The drawing under review shows one solid part. Ordinate dimensions are in mm from its lowest x, y, z. Round coordinates to 2 decimals unless told otherwise and drop trailing zeros. Write each loop counter-clockwise with the first axis right and the second up, starting at its lowest first coordinate (ties: lowest second). Pieces come first, ordered by that corner, then holes. Notation, with made-up numbers: (-5, -13) -> (44, -13) arc R30 cw to (44, 26) -> close; hole circle Ø7 at (-3, 3). An arc over 180 degrees is marked (long way). Write item = value, one per line. Start each with the question number.
Item 1: Add section B-B, the plane z = 150. State the section outline as (x, y) points.
Item 2: For pin 1 Ø13.5 at (x, z) = (20, 150) entering from -Y, flat-tipped, find the tip position at first contact; note if it passes through.
Item 3: To check wall thickness, follow L1, parallel to Z at x = 20, y = 5.25; L2, parallel to X at y = 4.5, z = 150; L3, parallel to Z at x = 13.5, y = 6.75. State the ranges of each line that lie inside material, in increasing order.
Item 4: Add section A-A, the plane x = 180. State the section outline as (y, z) points.
Item 5: Add section C-C, the plane y = 1.5. State the section outline as (x, z) points, then the cut area to 3 significant figures.
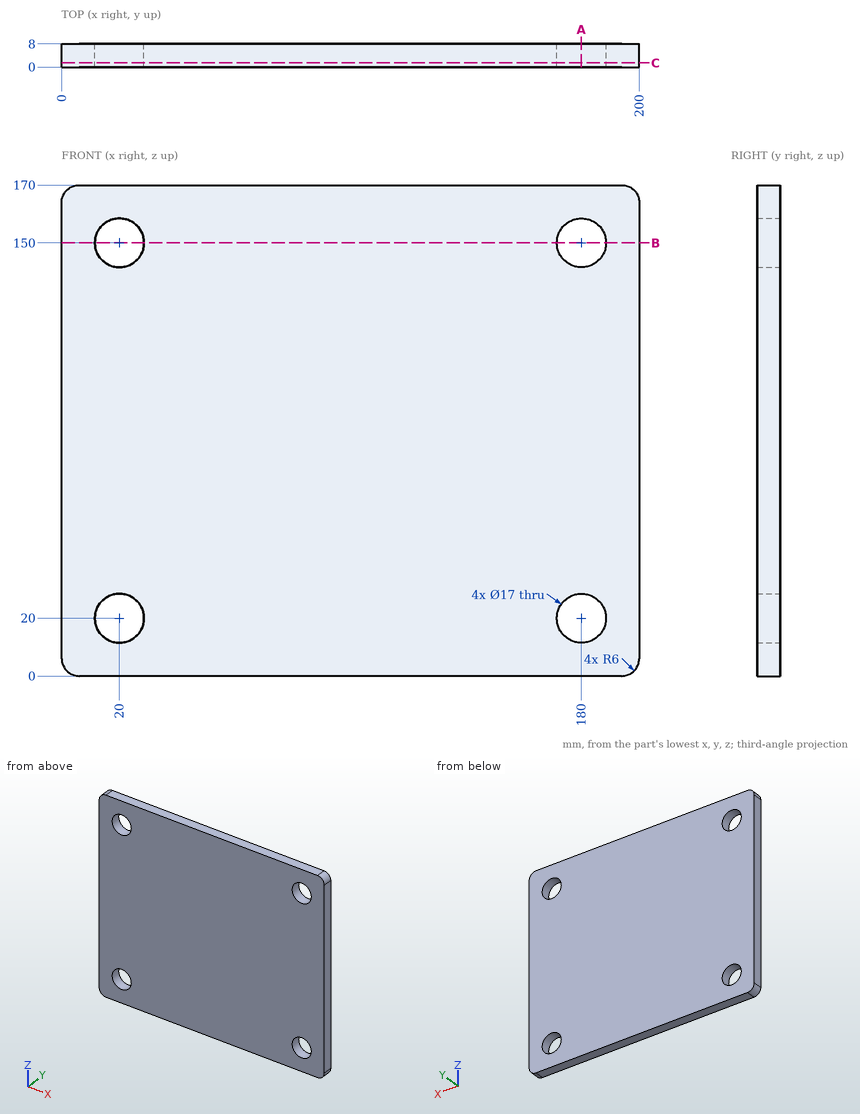
Result set:
q1.outline = (0, 0) -> (11.5, 0) -> (11.5, 8) -> (0, 8) -> close; (28.5, 0) -> (171.5, 0) -> (171.5, 8) -> (28.5, 8) -> close; (188.5, 0) -> (200, 0) -> (200, 8) -> (188.5, 8) -> close
q2.pin_1 = through
q3.L1 = 0 to 11.5, 28.5 to 141.5, 158.5 to 170
q3.L2 = 0 to 11.5, 28.5 to 171.5, 188.5 to 200
q3.L3 = 0 to 14.52, 25.48 to 144.52, 155.48 to 170
q4.outline = (0, 0) -> (8, 0) -> (8, 11.5) -> (0, 11.5) -> close; (0, 28.5) -> (8, 28.5) -> (8, 141.5) -> (0, 141.5) -> close; (0, 158.5) -> (8, 158.5) -> (8, 170) -> (0, 170) -> close
q5.outline = (0, 6) arc R6 ccw to (6, 0) -> (194, 0) arc R6 ccw to (200, 6) -> (200, 164) arc R6 ccw to (194, 170) -> (6, 170) arc R6 ccw to (0, 164) -> close; hole circle Ø17 at (20, 20); hole circle Ø17 at (20, 150); hole circle Ø17 at (180, 20); hole circle Ø17 at (180, 150)
q5.area = 33,100 mm²
